Read the model definition and answer for the solid it produces. Units are mm, in the model's axes. Give positions to 0.01 mm unless a question says otherwise; leave off trailing zeros. Order: outer loops, then holes, each group sorted by start corner. A loop starts at its lowest first (then second) coordinate and runs counter-clockwise, first axis right, second up. Notation, with made-up numbers: M -30,12 L 21,12 A17 ccw 21,29 Z; hole C -17.5,19 d8. An arc over 180 degrees is marked long. One line per item, written item: value.
from build123d import *

# Parameters (mm, degrees)
SKETCH1_R             = 11.1125
BOSS_EXTRUDE1_DEPTH   = 50.8
M3X0_5_TAPPED_HOLE1_D = 2.5


with BuildPart() as part:
    # Sketch1 → Boss-Extrude1 (new body)
    with BuildSketch(Plane(origin=(0, 0, 0), x_dir=(1, 0, 0), z_dir=(0, 1, 0))):
        Circle(SKETCH1_R)
    extrude(amount=BOSS_EXTRUDE1_DEPTH)

    # M3x0.5 Tapped Hole1 (through all)
    with Locations(Plane(origin=(0, 50.8, 0), x_dir=(1, 0, 0), z_dir=(0, 1, 0))):
        with Locations((0, 8), (6.92820323, 4), (6.92820323, -4), (0, -8), (-6.92820323, -4), (-6.92820323, 4)):
            Hole(M3X0_5_TAPPED_HOLE1_D / 2)


solid = part.part
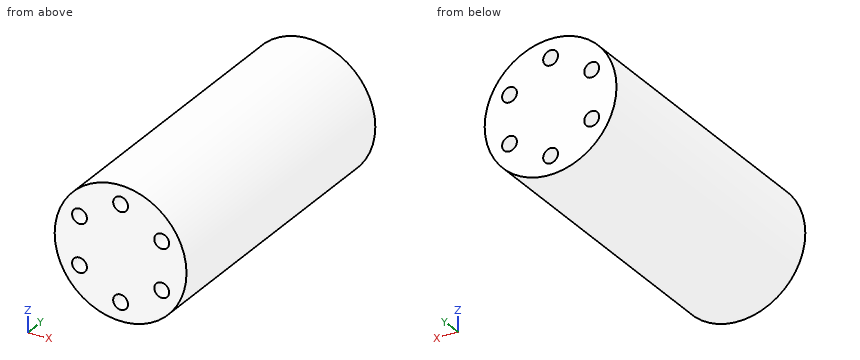
1) Each of these flat-tipped pins is pushed along its axis until it touches: pin 1 Ø10 at (y, z) = (31.5, 6) entering from +X; pin 2 Ø4 at (x, y) = (-3, 41) entering from +Z; pin 3 Ø10 at (x, y) = (-8, 6) entering from +Z. Where does it stop, or does it pass through?
Reported:
pin 1: stops at x = 11.07
pin 2: stops at z = 11.07
pin 3: stops at z = 10.7
2) Find section B-B, the plane y = 40.5. Count the separate pieces of the cut face and the enclosed holes in it, plus the area to 3 significant figures.
Reported:
separate pieces: 1
enclosed holes: 6
area: 358 mm^2
3) Find section D-D, the plane z = -8.5. Write down the section's boundary in (x, y).
Reported:
outline: M -7.16,0 L -1.15,0 L -1.15,50.8 L -7.16,50.8 Z; M 1.15,0 L 7.16,0 L 7.16,50.8 L 1.15,50.8 Z
4) Find section C-C, the plane z = -4. Write down the section's boundary in (x, y), plus the area to 3 significant figures.
Reported:
outline: M -10.37,0 L -8.18,0 L -8.18,50.8 L -10.37,50.8 Z; M -5.68,0 L 5.68,0 L 5.68,50.8 L -5.68,50.8 Z; M 8.18,0 L 10.37,0 L 10.37,50.8 L 8.18,50.8 Z
area: 799 mm^2
5) Consider probe 1 along Z at (x, y) = (-7.5, 48); probe 2 along Z at (x, y) = (-1, 29); probe 3 along X at (y, z) = (25, 4). Determine where each line is inside the solid, lowest interval first.
Reported:
probe 1: z = -8.2 to -5.11, -2.89 to 2.89, 5.11 to 8.2
probe 2: z = -11.07 to -8.75, -7.25 to 7.25, 8.75 to 11.07
probe 3: x = -10.37 to -8.18, -5.68 to 5.68, 8.18 to 10.37
6) Find section A-A, the plane x = 0. Write down the section's boundary in (y, z), plus the area to 3 significant figures.
Reported:
outline: M 0,-11.11 L 50.8,-11.11 L 50.8,-9.25 L 0,-9.25 Z; M 0,-6.75 L 50.8,-6.75 L 50.8,6.75 L 0,6.75 Z; M 0,9.25 L 50.8,9.25 L 50.8,11.11 L 0,11.11 Z
area: 875 mm^2
